Geometry check sheet. Reference: the model listing, model coordinates, mm. A direction names the side the tool comes from. Round coordinates to 2 decimals unless told otherwise and drop trailing zeros. Write each loop counter-clockwise with the first axis right and the second up, starting at its lowest first coordinate (ties: lowest second). Pieces come first, ordered by that corner, then holes. Notation, with made-up numbers: M 16.5,58.5 L 58.5,58.5 A25 cw 58.5,74.5 Z; hole C 10,-4.5 d1. An arc over 180 degrees is marked long. Answer in a Markdown table with one row per item. Add a question column.
from build123d import *

# Parameters (mm, degrees)
EXTRUDE_1_DEPTH     = 7
SKETCH_2_R          = 1.6
CUT_EXTRUDE_1_DEPTH = 2


with BuildPart() as part:
    # 草圖1 → 填料-伸長1 (new body)
    with BuildSketch(Plane.XY):
        Polygon((-13.5, 0), (13.5, 0), (13.5, -11), (18.5, -11), (18.5, -13), (11.5, -13), (11.5, -2), (-11.5, -2), (-11.5, -13), (-18.5, -13), (-18.5, -11), (-13.5, -11), align=None)
    extrude(amount=EXTRUDE_1_DEPTH)

    # 草圖2 → 除料-伸長1 (cut)
    with BuildSketch(Plane(origin=(0, -11, 0), x_dir=(1, 0, 0), z_dir=(0, 1, 0))):
        with Locations(Location((16, -3.5, 0), (0, 0, 270))):
            Circle(SKETCH_2_R)
        with Locations(Location((-16, -3.5, 0), (0, 0, 270))):
            Circle(SKETCH_2_R)
    extrude(amount=-CUT_EXTRUDE_1_DEPTH, mode=Mode.SUBTRACT)


solid = part.part
Item 1: Section check D-D, the plane z = 1.25. Record the boundary of the cut face in (x, y).
Item 2: Mould release check, pull along Z, two halves, no side actions. Record for faces 1 (the flat face through (11.5, -8, 3)), 2 (the flat face through (0.1, -1.7, 0)), 3 (the cylindrical face through (17.586, -11.986, 3.292)): +Z half, -Z half, draft (parallel to the pull), parting line (faces both ways), or undercut.
Item 3: Gauge pin test, flat ends, axial feed: pin 1 Ø1.5 at (x, z) = (3, 3.5) entering from -Y; pin 2 Ø2.5 at (x, z) = (-16.5, 3.5) entering from +Y; pin 3 Ø2 at (y, z) = (-1.5, 1.5) entering from -X. Record the tip position at first contact, or that the pin passes through.
Item 4: Section check C-C, the plane x = -16. Record the boundary of the cut face in (y, z).
Item 5: Section check A-A, the plane z = 3.5. Record the boundary of the cut face in (x, y), and give its area (3 significant figures).
Item 6: Scan lines: probe 1 along X at (y, z) = (-12.05, 3.5); probe 2 along X at (y, z) = (-8.25, 5.5); probe 3 along X at (y, z) = (-12.5, 6.5). Record each from-to range of solid material in increasing order. Write a range as from..to.
Item 7: Section check B-B, the plane y = -10.5. Record the boundary of the cut face in (x, z).
Item 8: Access from +Z, -Z, +X, -X, +Y, -Y to the whole of each face (thin tool, end or side, straight path). Record for faces 4 (the flat face through (0, -2, 3)), 5 (the flat face through (-17, -11, 2)), 6 (the flat face through (13.5, -5, 3)), 7 (the flat face through (0, 0, 3)).
Result sheet:
| question | item | result |
|---|---|---|
| 1 | outline | M -18.5,-13 L -11.5,-13 L -11.5,-2 L 11.5,-2 L 11.5,-13 L 18.5,-13 L 18.5,-11 L 13.5,-11 L 13.5,0 L -13.5,0 L -13.5,-11 L -18.5,-11 Z |
| 2 | face 1 | draft |
| 2 | face 2 | -Z half |
| 2 | face 3 | undercut |
| 3 | pin 1 | stops at y = -2 |
| 3 | pin 2 | stops at y = -11 |
| 3 | pin 3 | stops at x = -13.5 |
| 4 | outline | M -13,0 L -11,0 L -11,1.9 L -13,1.9 Z; M -13,5.1 L -11,5.1 L -11,7 L -13,7 Z |
| 5 | outline | M -18.5,-13 L -17.6,-13 L -17.6,-11 L -18.5,-11 Z; M -14.4,-13 L -11.5,-13 L -11.5,-2 L 11.5,-2 L 11.5,-13 L 14.4,-13 L 14.4,-11 L 13.5,-11 L 13.5,0 L -13.5,0 L -13.5,-11 L -14.4,-11 Z; M 17.6,-13 L 18.5,-13 L 18.5,-11 L 17.6,-11 Z |
| 5 | area | 105 mm^2 |
| 6 | probe 1 | x = -18.5..-17.6, -14.4..-11.5, 11.5..14.4, 17.6..18.5 |
| 6 | probe 2 | x = -13.5..-11.5, 11.5..13.5 |
| 6 | probe 3 | x = -18.5..-11.5, 11.5..18.5 |
| 7 | outline | M -13.5,0 L -11.5,0 L -11.5,7 L -13.5,7 Z; M 11.5,0 L 13.5,0 L 13.5,7 L 11.5,7 Z |
| 8 | face 4 | +Z, -Z, -Y |
| 8 | face 5 | +Z, -Z, -X, +Y |
| 8 | face 6 | +Z, -Z, +X, +Y |
| 8 | face 7 | +Z, -Z, +X, -X, +Y |
